Build history of the part. All positions in model axes, mm. Face numbers are marked on the shaded views. A direction names the side the tool comes from. Round coordinates to 2 decimals unless told otherwise and drop trailing zeros. Write each loop counter-clockwise with the first axis right and the second up, starting at its lowest first coordinate (ties: lowest second). Pieces come first, ordered by that corner, then holes. Notation, with made-up numbers: (50, 80) -> (101, 80) arc R23 cw to (101, 108) -> close; hole circle Ø7 at (77.25, 26). An arc over 180 degrees is marked (long way). Answer in a Markdown table with one row per item.
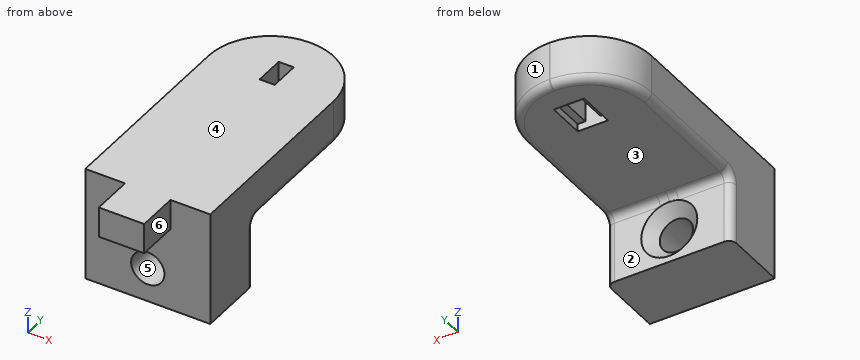
```python
from build123d import *

# Parameters (mm, degrees)
SKETCH1_W               = 16.5
SKETCH1_H               = 15
SKETCH1_R               = 2.2
BOSS_EXTRUDE1_DEPTH     = 9
CHAMFER1_SIZE           = 1.5
SKETCH2_W               = 16.5
SKETCH2_H               = 6
BOSS_EXTRUDE2_DEPTH     = 25
CUT_EXTRUDE2_DEPTH      = 37.125648783
CUT_EXTRUDE2_DEPTH_BACK = 37.125648783
SKETCH4_W               = 1
SKETCH4_H               = 4
SKETCH4_3_W             = 4
SKETCH4_3_H             = 6
SKETCH4_3_W_2           = 2
SKETCH4_3_H_2           = 4
CUT_EXTRUDE3_DEPTH      = 1
FILLET1_R               = 1
SKETCH7_W               = 4
SKETCH7_H               = 1
BOSS_EXTRUDE4_DEPTH     = 1
FILLET2_R               = 8.2
SKETCH8_W               = 6
SKETCH8_H               = 4
BOSS_EXTRUDE5_DEPTH     = 5.5


with BuildPart() as part:
    # Sketch1 → Boss-Extrude1 (new body)
    with BuildSketch(Plane(origin=(0, 0, 0), x_dir=(1, 0, 0), z_dir=(0, 1, 0))):
        Rectangle(SKETCH1_W, SKETCH1_H)
        with Locations(Location((0, 3, 0), (0, 0, 270))):
            Circle(SKETCH1_R, mode=Mode.SUBTRACT)
    extrude(amount=BOSS_EXTRUDE1_DEPTH)

    # Chamfer1
    chamfer1_edges = [part.edges().sort_by_distance(p)[0] for p in [
        (0, 9, -5.2),
    ]]
    chamfer(chamfer1_edges, length=CHAMFER1_SIZE)

    # Sketch2 → Boss-Extrude2 (add)
    with BuildSketch(Plane(origin=(0, 9, 0), x_dir=(1, 0, 0), z_dir=(0, 1, 0))):
        with Locations((0, -4.5)):
            Rectangle(SKETCH2_W, SKETCH2_H)
    extrude(amount=BOSS_EXTRUDE2_DEPTH)

    # Sketch4 → Cut-Extrude2 (cut, two sides: drawn at the far end of the back side and taken through both)
    with BuildSketch(Plane(origin=(0, 0, 1.5), x_dir=(-1, 0, 0), z_dir=(0, 0, -1)).offset(-CUT_EXTRUDE2_DEPTH_BACK)):
        with Locations((0.5, 27)):
            Rectangle(SKETCH4_W, SKETCH4_H)
        with Locations((-0.5, 27)):
            Rectangle(SKETCH4_W, SKETCH4_H)
    extrude(amount=CUT_EXTRUDE2_DEPTH + CUT_EXTRUDE2_DEPTH_BACK, mode=Mode.SUBTRACT)

    # Sketch4<3> → Cut-Extrude3 (cut)
    with BuildSketch(Plane(origin=(0, 0, 1.5), x_dir=(-1, 0, 0), z_dir=(0, 0, -1))):
        with Locations((0, 27)):
            Rectangle(SKETCH4_3_W, SKETCH4_3_H)
        with Locations((0, 27)):
            Rectangle(SKETCH4_3_W_2, SKETCH4_3_H_2, mode=Mode.SUBTRACT)
    extrude(amount=-CUT_EXTRUDE3_DEPTH, mode=Mode.SUBTRACT)

    # Fillet1
    fillet1_edges = [part.edges().sort_by_distance(p)[0] for p in [
        (-8.25, 9, -3),
        (8.25, 9, -3),
        (-8.25, 21.5, 1.5),
        (0, 9, 1.5),
        (8.25, 21.5, 1.5),
        (0, 34, 1.5),
    ]]
    fillet(fillet1_edges, radius=FILLET1_R)

    # Sketch7 → Boss-Extrude4 (add)
    with BuildSketch(Plane(origin=(0, 0, 2.5), x_dir=(-1, 0, 0), z_dir=(0, 0, -1))):
        with Locations((0, 24.5)):
            Rectangle(SKETCH7_W, SKETCH7_H)
    extrude(amount=BOSS_EXTRUDE4_DEPTH)

    # Fillet2
    # the kernel refuses this fillet: 8.2 mm, written as the material it takes off along each edge
    with BuildSketch(Plane(origin=(-0.05, 25.8, 1.5), x_dir=(-1, 0, 0), z_dir=(0, -1, 0))) as fillet2_piece_1:
        with BuildLine():
            CenterArc((7.2, -1), 1, 0, 90)
            Line((8.2, -1), (8.2, 0))
            Line((8.2, 0), (7.2, 0))
        make_face()
    revolve(axis=Axis((-0.05, 25.8, 1.5), (0, 0, -1)), revolution_arc=90, mode=Mode.SUBTRACT)
    with BuildSketch(Plane(origin=(0.05, 25.8, 1.5), x_dir=(0, 1, 0), z_dir=(-1, 0, 0))) as fillet2_piece_2:
        with BuildLine():
            CenterArc((7.2, -1), 1, 0, 90)
            Line((8.2, -1), (8.2, 0))
            Line((8.2, 0), (7.2, 0))
        make_face()
    revolve(axis=Axis((0.05, 25.8, 1.5), (0, 0, -1)), revolution_arc=90, mode=Mode.SUBTRACT)
    with BuildSketch(Plane(origin=(8.25, 34, 1.5), x_dir=(0, -1, 0), z_dir=(0, 0, 1)), Plane(origin=(-8.25, 34, 28), x_dir=(0, -1, 0), z_dir=(0, 0, -1))) as fillet2_piece_3:
        with BuildLine():
            CenterArc((FILLET2_R, -FILLET2_R), FILLET2_R, 90, 90)
            Line((0, -FILLET2_R), (0, 0))
            Line((0, 0), (FILLET2_R, 0))
        make_face()
    extrude(amount=26.5, mode=Mode.SUBTRACT)

    # Sketch8 → Boss-Extrude5 (add)
    with BuildSketch(Plane.XZ):
        with Locations((0, 5.5)):
            Rectangle(SKETCH8_W, SKETCH8_H)
    extrude(amount=BOSS_EXTRUDE5_DEPTH)


solid = part.part
```
Q1. Drop flat-ended pins along their axis: P1, Ø0.8, axis at y = 27, z = 2, coming from the -X side; P2, Ø3, axis at y = -3.5, z = 5, coming from the +X side; P3, Ø1.6, axis at x = -0.5, y = -2.5, coming from the -Z side. Give the stop position or say it passes through.
A:
| item | result |
|---|---|
| P1 | x = -8.18 |
| P2 | x = 3 |
| P3 | z = 3.5 |
Q2. Wall check: line 1 (X direction, y = 4.75, z = -3); line 2 (Y direction, x = 0.25, z = 6); line 3 (Z direction, x = -4.5, y = 28). Give the ranges that are in metal, low to high. Write a range as [from, to].
A:
| item | result |
|---|---|
| line 1 | [-8.25, -2.2], [2.2, 8.25] |
| line 2 | [-5.5, 25], [29, 34] |
| line 3 | [1.5, 7.5] |
Q3. Which spindle directions (+Z, -Z, +X, -X, +Y, -Y) get a long thin tool onto all of the face, cutting with end or side? Do the marked faces 1 and 2. Say none if no direction does.
A:
| item | result |
|---|---|
| face 1 | +Z, -Z, +X, +Y |
| face 2 | -Z, +X, -X, +Y |
Q4. Saw through at B-B on y = 7. Write the cut outline in (x, z).
A:
| item | result |
|---|---|
| outline | (-8.25, -7.5) -> (8.25, -7.5) -> (8.25, 7.5) -> (-8.25, 7.5) -> close; hole circle Ø4.4 at (0, -3) |
Q5. Saw through at C-C on z = 6.25. Write the cut outline in (x, y), plus the area to 3 significant figures.
A:
| item | result |
|---|---|
| outline | (-8.25, 0) -> (-3, 0) -> (-3, -5.5) -> (3, -5.5) -> (3, 0) -> (8.25, 0) -> (8.25, 25.8) arc R8.2 ccw to (0.05, 34) -> (-0.05, 34) arc R8.2 ccw to (-8.25, 25.8) -> close; hole (-1, 25) -> (1, 25) -> (1, 29) -> (-1, 29) -> close |
| area | 557 mm² |
Q6. Saw through at D-D on y = -2.5. Write the cut outline in (x, z).
A:
| item | result |
|---|---|
| outline | (-3, 3.5) -> (3, 3.5) -> (3, 7.5) -> (-3, 7.5) -> close |
Q7. Two-plate mould, pull along Z, no slides. Class the marked faces 3, 4, 5 and 6: released by +Z, released by -Z, zero draft, split by the parting line, or undercut.
A:
| item | result |
|---|---|
| face 3 | released by -Z |
| face 4 | released by +Z |
| face 5 | undercut |
| face 6 | zero draft |
Q8. Saw through at A-A on z = -3. Write the cut outline in (x, y).
A:
| item | result |
|---|---|
| outline | (-8.25, 0) -> (-2.2, 0) -> (-2.2, 7.5) -> (-3.7, 9) -> (-7.25, 9) arc R1 ccw to (-8.25, 8) -> close; (2.2, 0) -> (8.25, 0) -> (8.25, 8) arc R1 ccw to (7.25, 9) -> (3.7, 9) -> (2.2, 7.5) -> close |
